from build123d import *

# Parameters (mm, degrees)
SKETCH1_W           = 50
SKETCH1_H           = 4
BOSS_EXTRUDE1_DEPTH = 50
SKETCH2_R           = 13
CUT_EXTRUDE1_DEPTH  = 50
SKETCH4_R           = 2
CUT_EXTRUDE3_DEPTH  = 50
SKETCH7_W           = 4
SKETCH7_H           = 50
BOSS_EXTRUDE3_DEPTH = 20
SKETCH8_W           = 90
SKETCH8_H           = 4
BOSS_EXTRUDE4_DEPTH = 3
SKETCH9_W           = 25
SKETCH9_H           = 4
BOSS_EXTRUDE5_DEPTH = 4
FILLET1_R           = 10
SKETCH10_R          = 1.6
CUT_EXTRUDE4_DEPTH  = 20
CIRPATTERN1_COUNT   = 6
SKETCH11_R          = 6
CUT_EXTRUDE5_DEPTH  = 20
SKETCH12_W          = 4
SKETCH12_H          = 25
CUT_EXTRUDE6_DEPTH  = 20


with BuildPart() as part:
    # Sketch1 → Boss-Extrude1 (new body)
    with BuildSketch(Plane(origin=(0, 0, 0), x_dir=(1, 0, 0), z_dir=(0, 1, 0))):
        Rectangle(SKETCH1_W, SKETCH1_H)
    extrude(amount=BOSS_EXTRUDE1_DEPTH)

    # Sketch2 → Cut-Extrude1 (cut)
    with BuildSketch(Plane.XY.offset(2)):
        with Locations((0, 23)):
            Circle(SKETCH2_R)
    extrude(amount=-CUT_EXTRUDE1_DEPTH, mode=Mode.SUBTRACT)

    # Sketch4 → Cut-Extrude3 (cut)
    with BuildSketch(Plane.XY.offset(2)):
        with Locations((12.374368671, 35.374368671)):
            Circle(SKETCH4_R)
        with Locations((12.374368671, 10.625631329)):
            Circle(SKETCH4_R)
        with Locations((-12.374368671, 35.374368671)):
            Circle(SKETCH4_R)
        with Locations((-12.374368671, 10.625631329)):
            Circle(SKETCH4_R)
    extrude(amount=-CUT_EXTRUDE3_DEPTH, mode=Mode.SUBTRACT)

    # Sketch7 → Boss-Extrude3 (add)
    with BuildSketch(Plane.ZY.offset(25)):
        with Locations((0, 25)):
            Rectangle(SKETCH7_W, SKETCH7_H)
    boss_extrude3 = extrude(amount=BOSS_EXTRUDE3_DEPTH)

    # Mirror1: Boss-Extrude3 across plane
    add(boss_extrude3.mirror(Plane(origin=(0, 0, 0), x_dir=(0, 0, 1), z_dir=(1, 0, 0))))

    # Sketch8 → Boss-Extrude4 (add)
    with BuildSketch(Plane.XZ):
        Rectangle(SKETCH8_W, SKETCH8_H)
    extrude(amount=BOSS_EXTRUDE4_DEPTH)

    # Sketch9 → Boss-Extrude5 (add)
    with BuildSketch(Plane.XY.offset(2)):
        with Locations((-32.5, -5)):
            Rectangle(SKETCH9_W, SKETCH9_H)
        with Locations((32.5, -5)):
            Rectangle(SKETCH9_W, SKETCH9_H)
    extrude(amount=-BOSS_EXTRUDE5_DEPTH)

    # Fillet1
    fillet1_edges = [part.edges().sort_by_distance(p)[0] for p in [
        (-45, 50, 0),
        (45, 50, 0),
    ]]
    fillet(fillet1_edges, radius=FILLET1_R)

    # Sketch10 → Cut-Extrude4 (cut)
    with BuildSketch(Plane.XY.offset(2)):
        with Locations((-15.3, 23)):
            Circle(SKETCH10_R)
    cut_extrude4 = extrude(amount=-CUT_EXTRUDE4_DEPTH, mode=Mode.SUBTRACT)

    # CirPattern1: Cut-Extrude4 ×6 about axis
    cirpattern1_axis = Axis((0, 23, 0), (0, 0, 1))
    for i in range(1, CIRPATTERN1_COUNT):
        add(cut_extrude4.rotate(cirpattern1_axis, i * 360 / CIRPATTERN1_COUNT), mode=Mode.SUBTRACT)

    # Sketch11 → Cut-Extrude5 (cut)
    with BuildSketch(Plane.XY.offset(2)):
        with Locations((0, 15)):
            Circle(SKETCH11_R)
    extrude(amount=-CUT_EXTRUDE5_DEPTH, mode=Mode.SUBTRACT)

    # Sketch12 → Cut-Extrude6 (cut)
    with BuildSketch(Plane.XY.offset(2)):
        with Locations((43, 27.5)):
            Rectangle(SKETCH12_W, SKETCH12_H)
        with Locations((-43, 27.5)):
            Rectangle(SKETCH12_W, SKETCH12_H)
    extrude(amount=-CUT_EXTRUDE6_DEPTH, mode=Mode.SUBTRACT)


solid = part.part
Here's how the part is built. I have some questions about the finished solid (model axes, mm). A direction names the side the tool comes from. Coordinates: 2 decimals unless noted, no trailing zeros. Loops run counter-clockwise (first coordinate to the right, second up) from the corner with the lowest first, then second, coordinate; pieces in that order, holes last.
1. Imagine slicing it at C-C, the plane z = -1.35. Count the separate pieces of the cut face and the enclosed holes in it, and give its area (3 significant figures).
2. I need wall thicknesses on L1, parallel to Y at x = -9, z = -1.35; L2, parallel to X at y = 10, z = -1.55; L3, parallel to X at y = 36.5, z = 0.5. Which ranges of each line are inside material? Lowest first, please.
3. Imagine slicing it at D-D, the plane x = 0. Please give me the cut outline in (y, z).
4. Imagine slicing it at A-A, the plane x = 15.3. Please give me the cut outline in (y, z), and give its area (3 significant figures).
5. Imagine slicing it at B-B, the plane y = 23. Please give me the cut outline in (x, z).
6. If we mould it in two halves opening along Y, with no side actions, what happens to faces 1 (the flat face through (0, 50, 0)), 2 (the flat face through (9, 35, -2)), 3 (the cylindrical face through (14.28, 11.23, 0.03))? For each: pulls with the +Y half, pulls with the -Y half, needs draft (parallel to the pull), parting line crosses it, or undercut.
7. For faces 4 (the flat face through (32, -7, 0)), 5 (the flat face through (-41, 27, 0)), 6 (the flat face through (43, 15, 0)), which set-ups out of +Z, -Z, +X, -X, +Y, -Y let a thin tool reach every point of the face, with its end or its side?
8. For P1, Ø2.5, axis at x = -15.3, y = 23, coming from the +Z side; P2, Ø1.2, axis at x = -43.5, z = -0.5, coming from the +Y side, each with a flat end and sliding along its axis, tell me the tip position at first contact or that it passes through.
Taken from the geometry:
1. separate pieces: 1
1. enclosed holes: 11
1. area: 4,090 mm2
2. L1: y = -3 to 8.89, 10.61 to 13.62, 32.38 to 35.39, 37.11 to 50
2. L2: x = -45 to -14.27, -10.47 to -9.23, -6.07 to -3.32, 3.32 to 6.07, 9.23 to 10.47, 14.27 to 45
2. L3: x = -41 to -14.03, -10.72 to -9.23, -6.07 to 6.07, 9.23 to 10.72, 14.03 to 41
3. outline: (-3, -2) - (9, -2) - (9, 2) - (-3, 2) - close; (36, -2) - (50, -2) - (50, 2) - (36, 2) - close
4. outline: (-3, -2) - (21.4, -2) - (21.4, 2) - (-3, 2) - close; (24.6, -2) - (50, -2) - (50, 2) - (24.6, 2) - close
4. area: 199 mm2
5. outline: (-41, -2) - (-16.9, -2) - (-16.9, 2) - (-41, 2) - close; (-13.7, -2) - (-13, -2) - (-13, 2) - (-13.7, 2) - close; (13, -2) - (13.7, -2) - (13.7, 2) - (13, 2) - close; (16.9, -2) - (41, -2) - (41, 2) - (16.9, 2) - close
6. face 1: pulls with the +Y half
6. face 2: needs draft
6. face 3: undercut
7. face 4: +Z, -Z, +X, -X, -Y
7. face 5: +Z, -Z, -X
7. face 6: +Z, -Z, +X
8. P1: passes through
8. P2: stops at y = 46.13
